from build123d import *

# Parameters (mm, degrees)
F1_W     = 53.042872
F1_H     = 10.270788
F1_R     = 10.3251
F1_W_2   = 50.8
F1_H_2   = 6.999225
F2_DEPTH = 7.9375
F0_R     = 9.92251
F3_DEPTH = 88.9
F4_W     = 73.025
F4_H     = 36.5125
F5_DEPTH = 57.15


with BuildPart() as f2:
    # F1 (on Top) → F2 (new body)
    with BuildSketch(Plane.XY):
        with Locations((26.521436, 5.135394)):
            Rectangle(F1_W, F1_H)
        with BuildLine():
            Line((0, 10.270788), (53.042872, 10.270788))
            Line((53.042872, 10.270788), (53.042872, 19.05))
            ThreePointArc((53.042872, 19.05), (54.902744, 23.540128), (59.392872, 25.4))
            Line((59.392872, 25.4), (107.017872, 25.4))
            ThreePointArc((107.017872, 25.4), (129.214489, 48.74787), (104.775, 69.736539))
            Line((104.775, 69.736539), (57.15, 69.736539))
            ThreePointArc((57.15, 69.736539), (52.659872, 71.596411), (50.8, 76.086539))
            Line((50.8, 76.086539), (50.8, 81.900775))
            Line((50.8, 81.900775), (0, 81.900775))
            Line((0, 81.900775), (0, 10.270788))
        make_face()
        with Locations((68.917872, 47.824372)):
            Circle(F1_R, mode=Mode.SUBTRACT)
        with Locations((107.017872, 47.625)):
            Circle(F1_R, mode=Mode.SUBTRACT)
        with Locations((25.4, 85.400387)):
            Rectangle(F1_W_2, F1_H_2)
    extrude(amount=F2_DEPTH)

    # F0 (on Front) → F3 (join)
    with BuildSketch(Plane.XZ):
        with BuildLine():
            Line((0, 44.45), (0, 0))
            Line((0, 0), (57.15, 0))
            Line((57.15, 0), (57.15, 44.45))
            ThreePointArc((57.15, 44.45), (28.575, 73.025), (0, 44.45))
        make_face()
        with Locations((28.575, 44.45)):
            Circle(F0_R, mode=Mode.SUBTRACT)
    extrude(amount=-F3_DEPTH)

    # F4 (on face) → F5 (cut, through all)
    with BuildSketch(Plane.YZ.offset(57.15)):
        with Locations((44.45, 26.19375)):
            Rectangle(F4_W, F4_H)
    extrude(amount=-F5_DEPTH, mode=Mode.SUBTRACT)


solid = f2.part
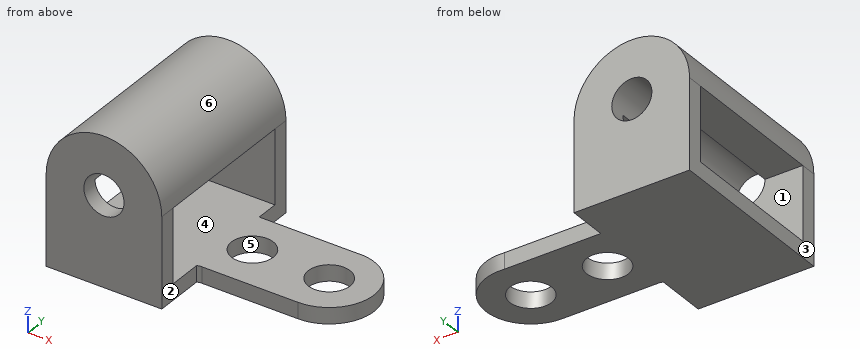
Geometry: final body of the model. Coordinates: model frame, mm. Face numbers are marked on the shaded views. A direction names the side the tool comes from. Give positions to 0.01 mm unless a question says otherwise; leave off trailing zeros. Order: outer loops, then holes, each group sorted by start corner. A loop starts at its lowest first (then second) coordinate and runs counter-clockwise, first axis right, second up. Notation, with made-up numbers: (-12, -9.75) -> (40, -9.75) arc R29 cw to (40, 28.25) -> close; hole circle Ø11 at (52.5, 54). An arc over 180 degrees is marked (long way). Put each result on its own line as item: value.
Q1. Reachability of the marked faces 1, 2 and 3 from +Z, -Z, +X, -X, +Y, -Y: full face, straight path, thin tool, end or side. Return the list, or none.
Here are the results:
face 1: +X, -X
face 2: +Z, -Z, +X, -Y
face 3: +Z, -Z, -X, +Y, -Y
Q2. Section C-C, the plane z = 41. Return loops of the section in (x, y).
Here are the results:
outline: (0, 0) -> (19.27, 0) -> (19.27, 7.94) -> (0, 7.94) -> close; (0, 80.96) -> (19.27, 80.96) -> (19.27, 88.9) -> (0, 88.9) -> close; (37.88, 0) -> (57.15, 0) -> (57.15, 7.94) -> (37.88, 7.94) -> close; (37.88, 80.96) -> (57.15, 80.96) -> (57.15, 88.9) -> (37.88, 88.9) -> close
Q3. Material intervals for L1, parallel to Y at x = 7, z = 32.5; L2, parallel to Y at x = 82, z = 6; L3, parallel to Z at x = 10.5, y = 70, sorted ascending.
Here are the results:
L1: y = 0 to 7.94, 80.96 to 88.9
L2: y = 25.4 to 69.74
L3: z = 0 to 7.94, 44.45 to 66.58
Q4. Section A-A, the plane z = 9.5. Return loops of the section in (x, y), then the cut area to 3 significant figures.
Here are the results:
outline: (0, 0) -> (57.15, 0) -> (57.15, 7.94) -> (0, 7.94) -> close; (0, 80.96) -> (57.15, 80.96) -> (57.15, 88.9) -> (0, 88.9) -> close
area: 907 mm^2
Q5. Pin query (flat end, axial travel): pin 1 (2.5 mm diameter, centred on x = 90.5, z = 4.5, fed in from -Y); pin 2 (1 mm diameter, centred on x = 50.5, y = 64, fed in from +Z); pin 3 (20 mm diameter, centred on y = 15.5, z = 29, fed in from +X); pin 4 (18 mm diameter, centred on x = 28.575, z = 44.45, fed in from -Y). Return the tip coordinate at first contact, or that it passes through.
Here are the results:
pin 1: stops at y = 25.4
pin 2: stops at z = 63.36
pin 3: stops at x = 57.15
pin 4: passes through
Q6. Draft query along X for the marked faces 4, 5 and 6. Return one class per face: released by +X, released by -X, zero draft, split by the parting line, or undercut.
Here are the results:
face 4: zero draft
face 5: undercut
face 6: split by the parting line
Q7. Section D-D, the plane y = 41.5. Count the separate pieces of the cut face and the enclosed holes in it, then the cut area to 3 significant figures.
Here are the results:
separate pieces: 4
enclosed holes: 0
area: 1,890 mm^2
